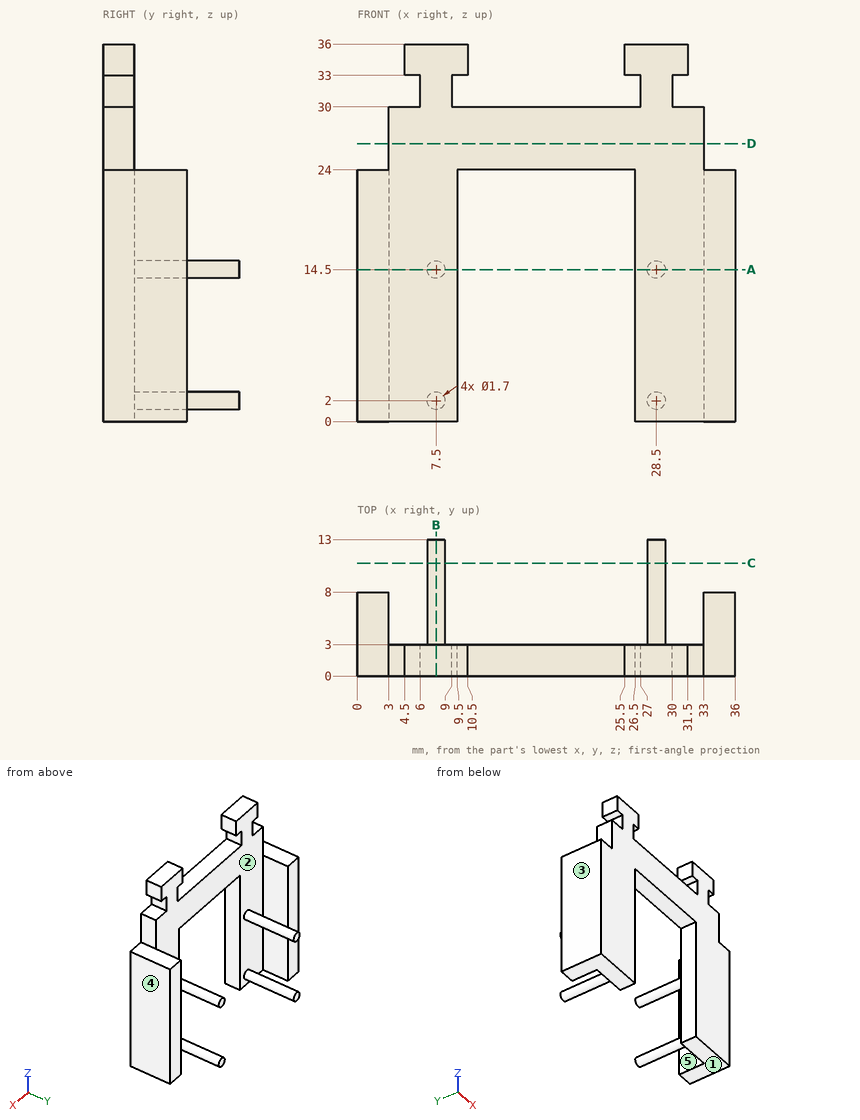
Design review of the part shown in the three views and the two pictorial views. Dimensions are in mm from the part's minimum x, y and z. A direction names the side the tool comes from. Coordinates: 2 decimals unless noted, no trailing zeros. Write each loop counter-clockwise with the first axis right and the second up, starting at its lowest first coordinate (ties: lowest second). Pieces come first, ordered by that corner, then holes.
(1) The part is to be moulded in two halves that separate along X. For the marked faces 1, 2 and 3, say which applies: +X half, -X half, draft (parallel to the pull), parting line (faces both ways), or undercut.
(2) Tool access review of the marked faces 4 and 5: name each direction out of +Z, -Z, +X, -X, +Y, -Y from which nothing blocks a thin tool from reaching the whole face with its end or side.
(3) Add section D-D on z = 26.5. Give the boundary of the cut face in (x, y).
(4) Add section C-C on y = 10.75. Give the boundary of the cut face in (x, z), then the cut area to 3 significant figures.
(5) Add section B-B on x = 7.5. Give the boundary of the cut face in (y, z).
(6) For pin 1 Ø1.5 at (y, z) = (2, 32) entering from +X; pin 2 Ø3.5 at (y, z) = (1, 31.5) entering from +X; pin 3 Ø1.5 at (x, y) = (2, 2.5) entering from +Z, all flat-tipped, find the tip position at first contact; note any pin that passes through.
(7) Wall thickness on probe 1 along X at (y, z) = (6.75, 5); probe 2 along X at (y, z) = (1.75, 18); probe 3 along Y at (x, z) = (8.5, 12.5): over which ranges is each line inside the solid? List them lowest first.
(8) Add section A-A on z = 14.5. Give the boundary of the cut face in (x, y), then the cut area to 3 significant figures.
Answer sheet:
1. face 1: draft
1. face 2: undercut
1. face 3: -X half
2. face 4: +Z, -Z, +X, +Y, -Y
2. face 5: +Z, -Z, +Y
3. outline: (3, 0) - (33, 0) - (33, 3) - (3, 3) - close
4. outline: circle Ø1.7 at (7.5, 2); circle Ø1.7 at (7.5, 14.5); circle Ø1.7 at (28.5, 2); circle Ø1.7 at (28.5, 14.5)
4. area: 9.08 mm2
5. outline: (0, 0) - (3, 0) - (3, 1.15) - (13, 1.15) - (13, 2.85) - (3, 2.85) - (3, 13.65) - (13, 13.65) - (13, 15.35) - (3, 15.35) - (3, 36) - (0, 36) - close
6. pin 1: stops at x = 30
6. pin 2: stops at x = 33
6. pin 3: stops at z = 24
7. probe 1: x = 0 to 3, 33 to 36
7. probe 2: x = 0 to 9.5, 26.5 to 36
7. probe 3: y = 0 to 3
8. outline: (0, 0) - (9.5, 0) - (9.5, 3) - (8.35, 3) - (8.35, 13) - (6.65, 13) - (6.65, 3) - (3, 3) - (3, 8) - (0, 8) - close; (26.5, 0) - (36, 0) - (36, 8) - (33, 8) - (33, 3) - (29.35, 3) - (29.35, 13) - (27.65, 13) - (27.65, 3) - (26.5, 3) - close
8. area: 121 mm2
